Can you work these out from the model? Positions are in its coordinate system, mm. Coordinates: 2 decimals unless noted, no trailing zeros. Order: outer loops, then holes, each group sorted by start corner. A loop starts at its lowest first (then second) coordinate and runs counter-clockwise, first axis right, second up.
```python
from build123d import *

# Parameters (mm, degrees)
SKETCH1_W               = 350
SKETCH1_H               = 200
BOSS_EXTRUDE1_DEPTH     = 11
SKETCH2_W               = 90
SKETCH2_H               = 30
SKETCH2_W_2             = 6
CUT_EXTRUDE1_DEPTH      = 1
CUT_EXTRUDE1_DEPTH_BACK = 12


with BuildPart() as part:
    # Sketch1 → Boss-Extrude1 (new body)
    with BuildSketch(Plane(origin=(0, 0, 0), x_dir=(1, 0, 0), z_dir=(0, 1, 0))):
        with Locations((32.608695652, -5.97826087)):
            Rectangle(SKETCH1_W, SKETCH1_H)
    extrude(amount=BOSS_EXTRUDE1_DEPTH)

    # Sketch2 → Cut-Extrude1 (cut, two sides)
    with BuildSketch(Plane(origin=(0, 11, 0), x_dir=(1, 0, 0), z_dir=(0, 1, 0))) as cut_extrude1_sk:
        with Locations((-73.391304348, -6.97826087)):
            Rectangle(SKETCH2_W, SKETCH2_H)
        with Locations((-129.391304348, -6.97826087)):
            Rectangle(SKETCH2_W_2, SKETCH2_H)
    extrude(amount=CUT_EXTRUDE1_DEPTH, mode=Mode.SUBTRACT)
    extrude(cut_extrude1_sk.sketch, amount=-CUT_EXTRUDE1_DEPTH_BACK, mode=Mode.SUBTRACT)


solid = part.part
```
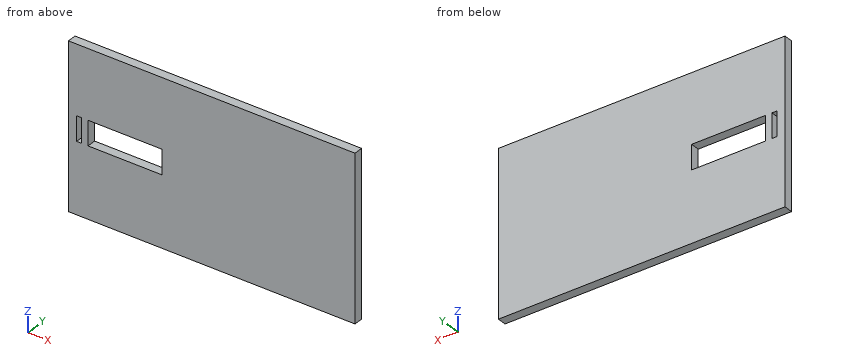
1. Imagine slicing it at B-B on z = 11. Please give me the cut outline in (x, y).
Completed:
outline: (-142.39, 0) - (-132.39, 0) - (-132.39, 11) - (-142.39, 11) - close; (-126.39, 0) - (-118.39, 0) - (-118.39, 11) - (-126.39, 11) - close; (-28.39, 0) - (207.61, 0) - (207.61, 11) - (-28.39, 11) - close
2. Imagine slicing it at C-C on y = 2.25. Please give me the cut outline in (x, z), then the cut area to 3 significant figures.
Completed:
outline: (-142.39, -94.02) - (207.61, -94.02) - (207.61, 105.98) - (-142.39, 105.98) - close; hole (-132.39, -8.02) - (-126.39, -8.02) - (-126.39, 21.98) - (-132.39, 21.98) - close; hole (-118.39, -8.02) - (-28.39, -8.02) - (-28.39, 21.98) - (-118.39, 21.98) - close
area: 67,100 mm2
3. Please list where these lines run through material, in increasing order: probe 1 along X at (y, z) = (7.5, -6.5); probe 2 along Z at (x, y) = (-87, 7.5).
Completed:
probe 1: x = -142.39 to -132.39, -126.39 to -118.39, -28.39 to 207.61
probe 2: z = -94.02 to -8.02, 21.98 to 105.98
4. Imagine slicing it at A-A on x = -66. Please give me the cut outline in (y, z).
Completed:
outline: (0, -94.02) - (11, -94.02) - (11, -8.02) - (0, -8.02) - close; (0, 21.98) - (11, 21.98) - (11, 105.98) - (0, 105.98) - close
